Check sheet for the modelled part. Datum: model origin and axes. Units: mm. A direction names the side the tool comes from. Give positions to 0.01 mm unless a question says otherwise; leave off trailing zeros. Write each loop counter-clockwise with the first axis right and the second up, starting at its lowest first coordinate (ties: lowest second). Pieces come first, ordered by that corner, then holes. Notation, with made-up numbers: (-25, 79.25) - (-7, 79.25) arc R17 cw to (-7, 101.25) - close; hole circle Ø10 at (-29.75, -11.75). An arc over 180 degrees is marked (long way). Return JSON: item names as keys, results as strings. Group by question number.
Autodesk Inventor part; units mm, degrees
ref_plane "YZ Plane" through (0, 0, 0) normal (1, 0, 0) x (0, 1, 0)
ref_plane "XZ Plane" through (0, 0, 0) normal (0, 1, 0) x (-1, 0, 0)
ref_plane "XY Plane" through (0, 0, 0) normal (0, 0, 1) x (1, 0, 0)
sketch "Sketch1" plane through (0, 0, 0) normal (0, 0, 1) x (1, 0, 0)
  line L0 (-12.5, -1.5) -> (12.5, -1.5)
  line L1 (12.5, -1.5) -> (12.5, 1.5)
  line L2 (12.5, 1.5) -> (-12.5, 1.5)
  line L3 (-12.5, 1.5) -> (-12.5, -1.5)
  line L4 (-12.5, -1.5) -> (12.5, 1.5) construction
  line L5 (12.5, -1.5) -> (-12.5, 1.5) construction
  line L6 (-5.6, 1.5) -> (-1.6, 1.5)
  line L7 (-1.6, 1.5) -> (-1.6, 10.5)
  line L8 (-1.6, 10.5) -> (-5.6, 10.5)
  line L9 (-5.6, 10.5) -> (-5.6, 1.5)
  line L10 (0, 1.5) -> (0, 12.2186)
  line L11 (1.6, 1.5) -> (1.6, 10.5)
  line L12 (1.6, 10.5) -> (5.6, 10.5)
  line L13 (5.6, 10.5) -> (5.6, 1.5)
  point P0 (0, 0)
  point P1 (5.6, 1.5)
  point P2 (1.6, 1.5)
  point P3 (-1.6, 1.5)
  dimension "d0" = 25
  dimension "d1" = 3
  dimension "d2" = 4
  dimension "d3" = 9
  dimension "d4" = 3.2
extrude "Extrusion1" add sketch "Sketch1" along normal blind 6.38
sketch "Sketch2" plane through (5.6, 1.5, 0) normal (0, 1, 0) x (1, 0, 0)
  circle A0 centre (3.9, -3.19) radius 1.5
  line L0 (6.9, 0) -> (6.9, -6.38)
  circle A1 centre (-15.1, -3.19) radius 1.5
  line L1 (-18.1, 0) -> (-18.1, -6.38)
  point P0 (-5.6, 0)
  dimension "d7" = 3
  dimension "d8" = 3
  dimension "d9" = 3
  dimension "d10" = 3
  dimension "d14" = 19
extrude "Extrusion2" cut sketch "Sketch2" against normal through all
fillet "Fillet1" radius 2 4 edges at (12.5, 0, 6.38) (12.5, 0, 0) (-12.5, 0, 6.38) (-12.5, 0, 0)
properties part number "Sensor"
Item 1: Material ranges on line 1 along X through (y, z) = (0.05, 3.19); line 2 along Z through (x, y) = (-9.5, 0); line 3 along X through (y, z) = (8.5, 5.5), recorded low to high. Write a range as from..to.
Item 2: Section check D-D on y = 0.5. Record the cut outline in (x, z), plus the area to 3 significant figures.
Item 3: Section check A-A on x = 9.5. Record the cut outline in (y, z), plus the area to 3 significant figures.
Item 4: Access from +Z, -Z, +X, -X, +Y, -Y to the whole of each face (thin tool, end or side, straight path). Record for faces 4 (the face through (-7, 1.5, 3)), 5 (the face through (0, 1.5, 3)), 6 (the face through (5.6, 6, 3)), 7 (the face through (12.5, 0, 3)), 8 (the face through (2, 3, 0)).
Item 5: Section check B-B on z = 3.19. Record the cut outline in (x, y), plus the area to 3 significant figures.
Item 6: Depth check by flat-ended pin: pin 1 (1.9 mm diameter, centred on y = 6, z = 4.5, fed in from +X); pin 2 (1.9 mm diameter, centred on y = 5.5, z = 3.5, fed in from -X); pin 3 (2.5 mm diameter, centred on x = -9.5, z = 3.19, fed in from -Y); pin 4 (1.9 mm diameter, centred on x = 9.5, z = 1.5, fed in from +Y). Enter the tip coordinate at first touch or a pass-through.
Item 7: Mould release check, pull along X, two halves, no side actions. Record for faces 1 (the face through (-10.69, 0.02, 4.1)), 2 (the face through (0, -1.5, 3)), 3 (the face through (11.93, 0.02, 0.6)): +X half, -X half, draft (parallel to the pull), parting line (faces both ways), or undercut.
Item 8: Section check C-C on y = 8. Record the cut outline in (x, z).
Reply:
{
 "1": {"line 1": "-12.5..-11, -8..8, 11..12.5", "line 2": "0..1.69, 4.69..6.38", "line 3": "-5.6..-1.6, 1.6..5.6"},
 "2": {"outline": "(-12.5, 2) arc R2 ccw to (-10.5, 0) - (10.5, 0) arc R2 ccw to (12.5, 2) - (12.5, 4.38) arc R2 ccw to (10.5, 6.38) - (-10.5, 6.38) arc R2 ccw to (-12.5, 4.38) - close; hole circle Ø3 at (-9.5, 3.19); hole circle Ø3 at (9.5, 3.19)", "area": "142 mm²"},
 "3": {"outline": "(-1.5, 0) - (1.5, 0) - (1.5, 1.69) - (-1.5, 1.69) - close; (-1.5, 4.69) - (1.5, 4.69) - (1.5, 6.38) - (-1.5, 6.38) - close", "area": "10.1 mm²"},
 "4": {"face 4": "+Z, -Z, -X, +Y", "face 5": "+Z, -Z, +Y", "face 6": "+Z, -Z, +X, +Y", "face 7": "+Z, -Z, +X, +Y, -Y", "face 8": "-Z, +X, -X, +Y, -Y"},
 "5": {"outline": "(-12.5, -1.5) - (-11, -1.5) - (-11, 1.5) - (-12.5, 1.5) - close; (-8, -1.5) - (8, -1.5) - (8, 1.5) - (5.6, 1.5) - (5.6, 10.5) - (1.6, 10.5) - (1.6, 1.5) - (-1.6, 1.5) - (-1.6, 10.5) - (-5.6, 10.5) - (-5.6, 1.5) - (-8, 1.5) - close; (11, -1.5) - (12.5, -1.5) - (12.5, 1.5) - (11, 1.5) - close", "area": "129 mm²"},
 "6": {"pin 1": "x = 5.6", "pin 2": "x = -5.6", "pin 3": "through", "pin 4": "y = 1.5"},
 "7": {"face 1": "undercut", "face 2": "draft", "face 3": "+X half"},
 "8": {"outline": "(-5.6, 0) - (-1.6, 0) - (-1.6, 6.38) - (-5.6, 6.38) - close; (1.6, 0) - (5.6, 0) - (5.6, 6.38) - (1.6, 6.38) - close"}
}
